```python
from build123d import *

# Parameters (mm, degrees)
F1_DEPTH = 55
F2_DEPTH = 15
F3_SIZE  = 2
F4_R     = 1.5
F5_DEPTH = 25
F6_W     = 6
F6_H     = 34
F7_DEPTH = 12.5
F8_R     = 1.5
F9_DEPTH = 12.5


with BuildPart() as f1:
    # F0 (on Top) → F1 (new body)
    with BuildSketch(Plane.XY):
        with BuildLine():
            ThreePointArc((2.5, -9.6824583655), (7.9056941504, -6.123724357), (10, 0))
            ThreePointArc((10, 0), (7.9056941504, 6.123724357), (2.5, 9.6824583655))
            Line((2.5, 9.6824583655), (2.5, -9.6824583655))
        make_face()
        with BuildLine():
            Line((2.5, -9.6824583655), (2.5, 9.6824583655))
            ThreePointArc((2.5, 9.6824583655), (0, 10), (-2.5, 9.6824583655))
            Line((-2.5, 9.6824583655), (-2.5, -9.6824583655))
            ThreePointArc((-2.5, -9.6824583655), (0, -10), (2.5, -9.6824583655))
        make_face()
        with BuildLine():
            Line((-2.5, -9.6824583655), (-2.5, 9.6824583655))
            ThreePointArc((-2.5, 9.6824583655), (-10, 0), (-2.5, -9.6824583655))
        make_face()
    extrude(amount=F1_DEPTH)

    # F0 (on Top) → F2 (join)
    with BuildSketch(Plane.XY):
        with BuildLine():
            Line((-2.5, -9.6824583655), (-2.5, 9.6824583655))
            ThreePointArc((-2.5, 9.6824583655), (-10, 0), (-2.5, -9.6824583655))
        make_face()
        with BuildLine():
            ThreePointArc((2.5, -9.6824583655), (7.9056941504, -6.123724357), (10, 0))
            ThreePointArc((10, 0), (7.9056941504, 6.123724357), (2.5, 9.6824583655))
            Line((2.5, 9.6824583655), (2.5, -9.6824583655))
        make_face()
    extrude(amount=-F2_DEPTH)

    # F3
    f3_edges = [f1.edges().sort_by_distance(p)[0] for p in [
        (2.5, -9.682458, 55),
    ]]
    chamfer(f3_edges, length=F3_SIZE)

    # F4 (on Right) → F5 (cut, symmetric)
    with BuildSketch(Plane.YZ):
        with Locations((0, -9.5)):
            Circle(F4_R)
    extrude(amount=F5_DEPTH, both=True, mode=Mode.SUBTRACT)

    # F6 (on Front) → F7 (cut, symmetric)
    with BuildSketch(Plane.XZ):
        with Locations((0, 23)):
            Rectangle(F6_W, F6_H)
    extrude(amount=F7_DEPTH, both=True, mode=Mode.SUBTRACT)

    # F8 (on Right) → F9 (cut, symmetric)
    with BuildSketch(Plane.YZ):
        with Locations((0, 19)):
            Circle(F8_R)
    extrude(amount=F9_DEPTH, both=True, mode=Mode.SUBTRACT)


solid = f1.part
```
Read the model definition and answer for the solid it produces. Units are mm, in the model's axes. A direction names the side the tool comes from. Round coordinates to 2 decimals unless told otherwise and drop trailing zeros. Write each loop counter-clockwise with the first axis right and the second up, starting at its lowest first coordinate (ties: lowest second). Pieces come first, ordered by that corner, then holes. Notation, with made-up numbers: (-0.75, -22) - (22.25, -22) arc R26 ccw to (22.25, 2) - close; hole circle Ø10 at (14, 14.5). An arc over 180 degrees is marked (long way). Use CSV: the item, a comma, the result in double quotes.
Q1. Determine the mould class of faces 4 (the flat face through (-2.5, 0, -7)), 5 (the flat face through (0, 0, 0)), 6 (the cylindrical face through (-6.452, -0.195, 20.487)) for opening direction Z: +Z half, -Z half, draft (parallel to the pull), parting line (faces both ways), or undercut.
Values:
face 4,"draft"
face 5,"-Z half"
face 6,"undercut"
Q2. Find section A-A, the plane z = 33.5. Write down the section's boundary in (x, y), then the cut area to 3 significant figures.
Values:
outline,"(-3, -9.54) - (-3, 9.54) arc R10 ccw to start; (3, -9.54) arc R10 ccw to (3, 9.54) - close"
area,"196 mm²"
Q3. Find section C-C, the plane z = -4. Write down the section's boundary in (x, y), then the cut area to 3 significant figures.
Values:
outline,"(-2.5, -9.68) - (-2.5, 9.68) arc R10 ccw to start; (2.5, -9.68) arc R10 ccw to (2.5, 9.68) - close"
area,"215 mm²"
Q4. Find section B-B, the plane z = 19. Write down the section's boundary in (x, y).
Values:
outline,"(-9.89, -1.5) arc R10 ccw to (-3, -9.54) - (-3, -1.5) - close; (-9.89, 1.5) - (-3, 1.5) - (-3, 9.54) arc R10 ccw to start; (3, -9.54) arc R10 ccw to (9.89, -1.5) - (3, -1.5) - close; (3, 1.5) - (9.89, 1.5) arc R10 ccw to (3, 9.54) - close"
Q5. Straight lines are drawn through the part: line 1 along Z through (x, y) = (5.5, 0); line 2 along Z through (x, y) = (0, -6.5); line 3 along X through (y, z) = (6, 14). For each, find the intervals that lie inside material, in ascending order.
Values:
line 1,"z = -15 to -11, -8 to 17.5, 20.5 to 55"
line 2,"z = 0 to 6, 40 to 55"
line 3,"x = -8 to -3, 3 to 8"
Q6. Each of these flat-tipped pins is pushed along its axis until it touches: pin 1 Ø2 at (x, z) = (-8, 16.5) entering from +Y; pin 2 Ø2 at (y, z) = (8, 15) entering from +X; pin 3 Ø3 at (x, y) = (0.5, 2.5) entering from -Z. Where does it stop, or does it pass through?
Values:
pin 1,"stops at y = 7.14"
pin 2,"stops at x = 7.14"
pin 3,"stops at z = 0"
Q7. A tool of negligible diameter and unlimited length cuts with its end or side. For faces 1 (the flat face through (0, 0, 40)), 2 (the flat face through (2.5, 0, -7)), 3 (the cylindrical face through (6.549, -0.195, 20.487)), from which of +Z, -Z, +X, -X, +Y, -Y can it reach the whole face along a straight path? Write none if from no direction.
Values:
face 1,"+Y, -Y"
face 2,"-Z, +Y, -Y"
face 3,"+X, -X"
Q8. Find section D-D, the plane x = 7. Count the separate pieces of the cut face and the enclosed holes in it, then the cut area to 3 significant figures.
Values:
separate pieces,"1"
enclosed holes,"2"
area,"980 mm²"
